Autodesk Inventor part; units mm, degrees
ref_plane "YZ Plane" through (0, 0, 0) normal (1, 0, 0) x (0, 1, 0)
ref_plane "XZ Plane" through (0, 0, 0) normal (0, 1, 0) x (-1, 0, 0)
ref_plane "XY Plane" through (0, 0, 0) normal (0, 0, 1) x (1, 0, 0)
sketch "Sketch1" plane through (0, 0, 0) normal (0, 1, 0) x (-1, 0, 0)
  line L0 (-38.6259, 0.7937) -> (38.6259, 0.7937)
  line L1 (-38.1254, -0.7938) -> (-38.6259, 0.7937) construction
  line L2 (-38.6259, 0.7937) -> (-59.8424, -14.0622)
  line L3 (-59.8424, -14.0622) -> (-58.9319, -15.3626)
  line L4 (-58.9319, -15.3626) -> (-38.1254, -0.7938)
  line L5 (-38.1254, -0.7938) -> (38.1254, -0.7938)
  line L6 (38.1254, -0.7938) -> (56.6432, -13.76)
  line L7 (56.6432, -13.76) -> (57.5537, -12.4596)
  line L8 (57.5537, -12.4596) -> (38.6259, 0.7937)
  point P0 (0, 0)
  dimension "d75" = 1.5875
  dimension "d76" = 1.5875
  dimension "d77" = 1.5875
  dimension "d78" = 145
  dimension "d79" = 76.2508
  dimension "d80" = 38.1254
  dimension "d81" = 0.7937
  dimension "d82" = 145
  dimension "d83" = 22.606
  dimension "d84" = 25.4
extrude "Extrusion1" add sketch "Sketch1" along normal blind 109.855
sketch "Sketch3" plane through (38.1254, 0, -0.7938) normal (0, 0, -1) x (-1, 0, 0)
  line L0 (38.1254, 97.0628) -> (38.1254, 73.759) construction
  line L1 (76.2508, 0) -> (76.2508, 109.855) construction
  line L2 (0, 0) -> (0, 109.855) construction
  line L3 (76.7513, 109.855) -> (-0.5005, 109.855) construction
  point P0 (38.1254, 0)
  point P1 (12.7254, 106.68)
  point P2 (63.5254, 106.68)
  dimension "d85" = 76.2508
  dimension "d86" = 38.1254
  dimension "d87" = 25.4
  dimension "d88" = 3.175
  dimension "d93" = 50.8
hole "Hole1" at (25.4, 106.68, -0.7938) at (-25.4, 106.68, -0.7938) direction (0, 0, 1) diameter 3.2766 end through all
sketch "Sketch4" plane through (-38.6259, 0, 0.7937) normal (0, 0, 1) x (1, 0, 0)
  line L0 (0, 0) -> (0, 109.855)
  line L1 (77.2519, 0) -> (0, 0)
  line L2 (77.2519, 0) -> (77.2519, 109.855)
  point P0 (38.6259, 0)
  point P1 (69.3017, 9.5758)
  point P2 (7.9502, 22.5806)
  point P3 (7.9502, 9.5758)
  point P4 (69.3017, 22.5806)
  dimension "d112" = 7.9502
  dimension "d113" = 9.5758
  dimension "d114" = 9.5758
  dimension "d115" = 7.9502
  dimension "d116" = 7.9502
  dimension "d117" = 7.9502
  dimension "d118" = 22.5806
  dimension "d119" = 22.5806
hole "Hole3" at (30.6757, 9.5758, 0.7937) at (-30.6757, 22.5806, 0.7937) at (-30.6757, 9.5758, 0.7937) at (30.6757, 22.5806, 0.7937) direction (0, 0, -1) diameter 2.8448 end through all
equation "\"d75\" = d77"
equation "\"d76\" = d77"
equation "\"d86\" = 0.5 * d85"
properties part number "solar sheild" material "Aluminum 6061"
Geometry check sheet. Reference: the model listing, model coordinates, mm. A direction names the side the tool comes from. Round coordinates to 2 decimals unless told otherwise and drop trailing zeros. Loops run counter-clockwise (first coordinate to the right, second up) from the corner with the lowest first, then second, coordinate; pieces in that order, holes last. Notation, with made-up numbers: (4, 61.25) -> (35, 61.25) arc R23 ccw to (35, 91.25) -> close; hole circle Ø8 at (42, -25.5). An arc over 180 degrees is marked (long way). Answer as a JSON object with one key per item and string values. Group by question number.
Item 1: Cross-section at C-C, the plane z = -4.5. Record the cut outline in (x, y) (3 decimals), plus the area to 3 significant figures.
Item 2: Release check for a two-part mould opening along Y. For faces 3 (the face through (1, 0, 0)), 4 (the face through (-32.086, 22.766, -0.011)), 5 (the face through (48.7, 54.2, -8.2)), 6 (the face through (1, 109.855, 0)) record: pulls with the +Y half, pulls with the -Y half, needs draft (parallel to the pull), parting line crosses it, or undercut.
Item 3: Cross-section at A-A, the plane x = -25.4. Record the cut outline in (y, z) (3 decimals), plus the area to 3 significant figures.
Item 4: Depth check by flat-ended pin: pin 1 Ø5 at (x, y) = (43, 46) entering from +Z; pin 2 Ø1.5 at (y, z) = (26, -3) entering from +X (3 decimals); pin 3 Ø6 at (y, z) = (60, -2) entering from -X. Enter the tip coordinate at first touch or a pass-through.
Item 5: Cross-section at B-B, the plane y = 106.68. Record the cut outline in (x, z).
Item 6: Thickness scan on line 1 along Y through (x, z) = (-25.4, -0.4) (3 decimals); line 2 along X through (y, z) = (106.68, -0.4); line 3 along X through (y, z) = (26, -11.75). Record the ranges inside material, lowest first.
Item 7: Set-up check for faces 1 (the face through (-25.892, 108.243, 0.011)), 2 (the face through (-47.255, 54.159, -7.186)): record each of +Z, -Z, +X, -X, +Y, -Y from which the full face is reachable in a straight line by a thin tool's end or side.
Item 8: Cross-section at D-D, the plane y = 73.5. Record the cut outline in (x, z).
Determined:
{
 "1": {"outline": "(-46.186, 0) -> (-43.418, 0) -> (-43.418, 109.855) -> (-46.186, 109.855) -> close; (43.418, 0) -> (46.186, 0) -> (46.186, 109.855) -> (43.418, 109.855) -> close", "area": "608 mm²"},
 "2": {"face 3": "pulls with the -Y half", "face 4": "undercut", "face 5": "needs draft", "face 6": "pulls with the +Y half"},
 "3": {"outline": "(0, -0.794) -> (105.042, -0.794) -> (105.042, 0.794) -> (0, 0.794) -> close; (108.318, -0.794) -> (109.855, -0.794) -> (109.855, 0.794) -> (108.318, 0.794) -> close", "area": "169 mm²"},
 "4": {"pin 1": "stops at z = -0.52", "pin 2": "stops at x = 45.115", "pin 3": "stops at x = -46.9"},
 "5": {"outline": "(-57.55, -12.46) -> (-56.64, -13.76) -> (-38.13, -0.79) -> (-27.04, -0.79) -> (-27.04, 0.79) -> (-38.63, 0.79) -> close; (-23.76, -0.79) -> (23.76, -0.79) -> (23.76, 0.79) -> (-23.76, 0.79) -> close; (27.04, -0.79) -> (38.13, -0.79) -> (58.93, -15.36) -> (59.84, -14.06) -> (38.63, 0.79) -> (27.04, 0.79) -> close"},
 "6": {"line 1": "y = 0 to 105.042, 108.318 to 109.855", "line 2": "x = -40.33 to -27.04, -23.76 to 23.76, 27.04 to 40.33", "line 3": "x = -56.54 to -53.77, 53.77 to 56.54"},
 "7": {"face 1": "+Z, -Z", "face 2": "-Z, +Y, -Y"},
 "8": {"outline": "(-57.55, -12.46) -> (-56.64, -13.76) -> (-38.13, -0.79) -> (38.13, -0.79) -> (58.93, -15.36) -> (59.84, -14.06) -> (38.63, 0.79) -> (-38.63, 0.79) -> close"}
}
